Check sheet for the modelled part. Datum: model origin and axes. Units: mm. A direction names the side the tool comes from. Give positions to 0.01 mm unless a question says otherwise; leave off trailing zeros. Order: outer loops, then holes, each group sorted by start corner. A loop starts at its lowest first (then second) coordinate and runs counter-clockwise, first axis right, second up. Notation, with made-up numbers: M -11.5,-40 L 33.5,-40 A8 cw 33.5,-35 Z; hole C 62.25,32.5 d4. An arc over 180 degrees is marked long. Answer in a Markdown table with one row per item. Add a question column.
from build123d import *

# Parameters (mm, degrees)
SKETCH1_3_R         = 1.5
SKETCH1_3_R_2       = 2
SKETCH1_3_W         = 2.5
SKETCH1_3_H         = 20
BOSS_EXTRUDE2_DEPTH = 1.25
FILLET2_R           = 10


with BuildPart() as part:
    # Sketch1_3 → Boss-Extrude2 (new, symmetric)
    with BuildSketch(Plane.XY):
        Polygon((48.5, 37.5), (-48.5, 37.5), (-48.5, -12.5), (-25, -37.5), (25, -37.5), (48.5, -12.5), align=None)
        with Locations((0, -29.5)):
            Circle(SKETCH1_3_R, mode=Mode.SUBTRACT)
        with Locations((-16.5, -27.75)):
            Circle(SKETCH1_3_R, mode=Mode.SUBTRACT)
        with Locations((16.5, -27.75)):
            Circle(SKETCH1_3_R, mode=Mode.SUBTRACT)
        with Locations((-35.566666667, 27.5)):
            Circle(SKETCH1_3_R, mode=Mode.SUBTRACT)
        with Locations((35.566666667, 27.5)):
            Circle(SKETCH1_3_R, mode=Mode.SUBTRACT)
        with Locations((-16.5, -2.75)):
            Circle(SKETCH1_3_R_2, mode=Mode.SUBTRACT)
        with Locations((16.5, -2.75)):
            Circle(SKETCH1_3_R_2, mode=Mode.SUBTRACT)
        with Locations((-45.25, 12.5)):
            Rectangle(SKETCH1_3_W, SKETCH1_3_H, mode=Mode.SUBTRACT)
        with Locations((45.25, 12.5)):
            Rectangle(SKETCH1_3_W, SKETCH1_3_H, mode=Mode.SUBTRACT)
    extrude(amount=BOSS_EXTRUDE2_DEPTH, both=True)

    # Fillet2
    fillet2_edges = [part.edges().sort_by_distance(p)[0] for p in [
        (48.5, -12.5, 0),
        (25, -37.5, 0),
        (-25, -37.5, 0),
        (-48.5, -12.5, 0),
    ]]
    fillet(fillet2_edges, radius=FILLET2_R)


solid = part.part
Q1. Cross-section at A-A (y = 5.5). Record the boundary of the cut face in (x, z).
Q2. Cross-section at D-D (x = 29). Record the boundary of the cut face in (y, z), and give its area (3 significant figures).
Q3. Go/stop test with flat-tipped pins: pin 1 (1 mm diameter, centred on y = -27.5, z = 0.5, fed in from +X); pin 2 (1.8 mm diameter, centred on x = 0, y = -29.5, fed in from -Z). Record where each tip stops, or that it passes through.
Q4. Tool access check on faces 5 (the flat face through (45, 2.5, 0)), 6 (the flat face through (-36.999, -24.735, 0.018)). Record the directions out of +Z, -Z, +X, -X, +Y, -Y that give a thin tool (end or side, any length) a straight path to the whole face; none if there is none.
Q5. Draft check along X on faces 1 (the flat face through (36.75, -25, 0.02)), 2 (the cylindrical face through (-47.777, -12.27, 0.018)), 3 (the flat face through (-45, 22.5, 0)), 4 (the flat face through (-1, 1, 1.25)). Enter one of: pulls with the +X half, pulls with the -X half, needs draft (parallel to the pull), parting line crosses it, or undercut.
Q6. Cross-section at B-B (x = -16.5). Record the boundary of the cut face in (y, z), and give its area (3 significant figures).
Q7. Cross-section at C-C (z = -0.3). State how many separate pieces and enclosed holes the cut face has, and give its area (3 significant figures).
Q8. Thickness scan on probe 1 along X at (y, z) = (-2.5, -0.95); probe 2 along X at (y, z) = (6, -0.55); probe 3 along Y at (x, z) = (-21, 0.4). Record the ranges inside material, lowest first.
Values follow:
| question | item | result |
|---|---|---|
| 1 | outline | M -48.5,-1.25 L -46.5,-1.25 L -46.5,1.25 L -48.5,1.25 Z; M -44,-1.25 L 44,-1.25 L 44,1.25 L -44,1.25 Z; M 46.5,-1.25 L 48.5,-1.25 L 48.5,1.25 L 46.5,1.25 Z |
| 2 | outline | M -33.24,-1.25 L 37.5,-1.25 L 37.5,1.25 L -33.24,1.25 Z |
| 2 | area | 177 mm² |
| 3 | pin 1 | x = 34.87 |
| 3 | pin 2 | through |
| 4 | face 5 | +Z, -Z |
| 4 | face 6 | +Z, -Z, -X, -Y |
| 5 | face 1 | pulls with the +X half |
| 5 | face 2 | pulls with the -X half |
| 5 | face 3 | undercut |
| 5 | face 4 | needs draft |
| 6 | outline | M -37.5,-1.25 L -29.25,-1.25 L -29.25,1.25 L -37.5,1.25 Z; M -26.25,-1.25 L -4.75,-1.25 L -4.75,1.25 L -26.25,1.25 Z; M -0.75,-1.25 L 37.5,-1.25 L 37.5,1.25 L -0.75,1.25 Z |
| 6 | area | 170 mm² |
| 7 | separate pieces | 1 |
| 7 | enclosed holes | 9 |
| 7 | area | 6,520 mm² |
| 8 | probe 1 | -48.5 to -18.48, -14.52 to 14.52, 18.48 to 48.5 |
| 8 | probe 2 | -48.5 to -46.5, -44 to 44, 46.5 to 48.5 |
| 8 | probe 3 | -37.49 to 37.5 |
